from build123d import *

# Parameters (mm, degrees)
HOLE_WIZARD_M4_1_D = 3.3


with BuildPart() as part:
    # 草图1 → 旋转1 (revolve)
    with BuildSketch(Plane.XY, mode=Mode.PRIVATE) as revolve_1_sk:
        Polygon((41.5, 9), (46, 9), (46, 6.5), (53, 6.5), (53, 2.5), (46, 2.5), (46, 0), (43, 0), (43, 8), (41.5, 8), align=None)
    revolve(revolve_1_sk.sketch.rotate(Axis((0, 0, 0), (0, 1, 0)), 90), axis=Axis((0, 0, 0), (0, 1, 0)))

    # M4 螺纹孔1 (through all)
    with Locations(Plane(origin=(0, 2.5, 0), x_dir=(-1, 0, 0), z_dir=(0, -1, 0))):
        with Locations((-35.001785669, 35.001785669), (35.001785669, 35.001785669), (35.001785669, -35.001785669), (-35.001785669, -35.001785669)):
            Hole(HOLE_WIZARD_M4_1_D / 2)


solid = part.part
Model file for the job. Use its own axes, mm. A direction names the side the tool comes from. Coordinates: 2 decimals unless noted, no trailing zeros. Write each loop counter-clockwise with the first axis right and the second up, starting at its lowest first coordinate (ties: lowest second). Pieces come first, ordered by that corner, then holes. Notation, with made-up numbers: (80.5, -23) -> (116.5, -23) arc R29 ccw to (116.5, 6) -> close; hole circle Ø11 at (79, 12). An arc over 180 degrees is marked (long way). One line per item, written item: value. Start each with the question number.
1) Which spindle directions (+Z, -Z, +X, -X, +Y, -Y) get a long thin tool onto all of the face, cutting with end or side? Do faces 1 (the face through (-45.61, 7.73, 5.99)), 2 (the face through (-34.24, 4.528, 36.466)), 3 (the face through (-35.2, 8, 22.5)). Say none if no direction does.
2) Slice it at B-B on x = 0. Write the cut outline in (y, z).
3) Probe probe 1 along Z at (x, y) = (35, 2.75); probe 2 along Y at (x, z) = (16.5, 39); probe 3 along Z at (x, y) = (11, 8.25). List the from-to ranges inside material, lowest first.
4) Slice it at A-A on z = 0. Write the cut outline in (x, y).
5) Pull direction X, two halves, no side cores. Call faces 4 (the face through (-34.11, 4.53, -36.39)), 5 (the face through (-16, 2.5, 43.4)), 6 (the face through (-45.61, 1.23, 5.99)): +X half, -X half, draft (parallel to the pull), parting line (faces both ways), or undercut.
6) Flat gauge pins, fed straight in: pin 1 Ø1.5 at (y, z) = (8, -36) entering from +X; pin 2 Ø5.5 at (x, z) = (-35, 35) entering from -Y; pin 3 Ø2 at (y, z) = (3.5, 26) entering from +X. Where does each tip first touch, or does it go through?
Answers follow:
1. face 1: +Y
1. face 2: +Y, -Y
1. face 3: -Y
2. outline: (0, -46) -> (2.5, -46) -> (2.5, -53) -> (6.5, -53) -> (6.5, -46) -> (9, -46) -> (9, -41.5) -> (8, -41.5) -> (8, -43) -> (0, -43) -> close; (0, 43) -> (8, 43) -> (8, 41.5) -> (9, 41.5) -> (9, 46) -> (6.5, 46) -> (6.5, 53) -> (2.5, 53) -> (2.5, 46) -> (0, 46) -> close
3. probe 1: -39.8 to -36.65, -33.35 to -24.98, 24.98 to 33.35, 36.65 to 39.8
3. probe 2: 8 to 9
3. probe 3: -44.67 to -40.02, 40.02 to 44.67
4. outline: (-53, 2.5) -> (-46, 2.5) -> (-46, 0) -> (-43, 0) -> (-43, 8) -> (-41.5, 8) -> (-41.5, 9) -> (-46, 9) -> (-46, 6.5) -> (-53, 6.5) -> close; (41.5, 8) -> (43, 8) -> (43, 0) -> (46, 0) -> (46, 2.5) -> (53, 2.5) -> (53, 6.5) -> (46, 6.5) -> (46, 9) -> (41.5, 9) -> close
5. face 4: undercut
5. face 5: draft
5. face 6: parting line
6. pin 1: x = 29.55
6. pin 2: y = 2.5
6. pin 3: x = 46.73
